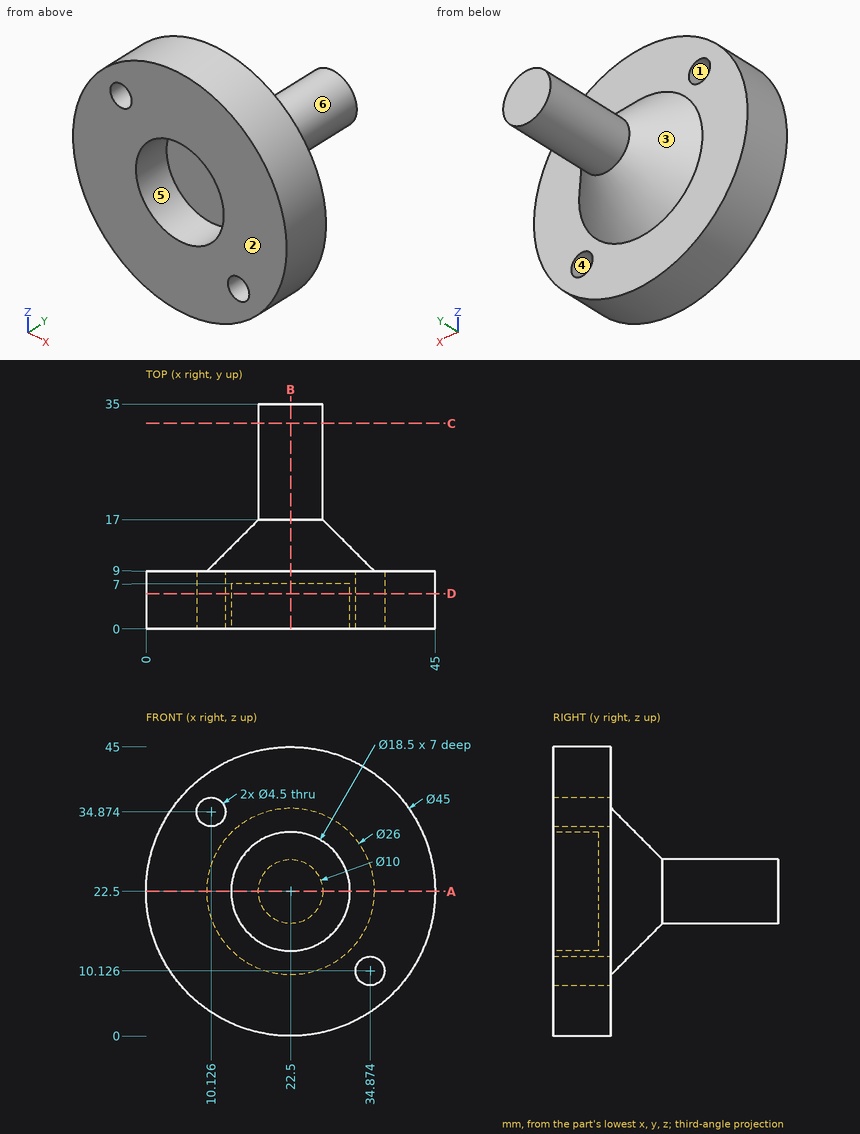
The drawing under review shows one solid part. Ordinate dimensions are in mm from its lowest x, y, z. A direction names the side the tool comes from. Round coordinates to 2 decimals unless told otherwise and drop trailing zeros. Loops run counter-clockwise (first coordinate to the right, second up) from the corner with the lowest first, then second, coordinate; pieces in that order, holes last. Notation, with made-up numbers: (-25.75, 1.25) -> (28.25, 1.25) arc R29 ccw to (28.25, 21.25) -> close; hole circle Ø8 at (-30.5, 70). An arc over 180 degrees is marked (long way). Answer in a Markdown table with one row per item.
1) For pin 1 Ø1 at (x, z) = (21, 9.5) entering from +Y (1 decimal); pin 2 Ø9 at (x, z) = (25, 26) entering from -Y; pin 3 Ø1.5 at (x, y) = (17.5, 17.5) entering from -Z (1 decimal), all flat-tipped, find the tip position at first contact; note any pin that passes through.
Taken from the geometry:
| item | result |
|---|---|
| pin 1 | stops at y = 9.4 |
| pin 2 | stops at y = 7 |
| pin 3 | stops at z = 19.9 |
2) Consider section C-C, the plane y = 32. Write out the cut boundary in (x, z).
Taken from the geometry:
| item | result |
|---|---|
| outline | circle Ø10 at (22.5, 22.5) |
3) Consider section B-B, the plane x = 22.5. Write out the cut boundary in (y, z).
Taken from the geometry:
| item | result |
|---|---|
| outline | (0, 0) -> (9, 0) -> (9, 9.5) -> (17, 17.5) -> (35, 17.5) -> (35, 27.5) -> (17, 27.5) -> (9, 35.5) -> (9, 45) -> (0, 45) -> (0, 31.75) -> (7, 31.75) -> (7, 13.25) -> (0, 13.25) -> close |
4) Draft analysis for pull direction X (two halves, no side actions). For the marked faces 1, 2 and 3, state which applies: pulls with the +X half, pulls with the -X half, needs draft (parallel to the pull), parting line crosses it, or undercut.
Taken from the geometry:
| item | result |
|---|---|
| face 1 | undercut |
| face 2 | needs draft |
| face 3 | parting line crosses it |
5) Consider section D-D, the plane y = 5.5. Count the separate pieces of the cut face and the enclosed holes in it, plus the area to 3 significant figures.
Taken from the geometry:
| item | result |
|---|---|
| separate pieces | 1 |
| enclosed holes | 3 |
| area | 1,290 mm² |
6) Consider section A-A, the plane z = 22.5. Write out the cut boundary in (x, y).
Taken from the geometry:
| item | result |
|---|---|
| outline | (0, 0) -> (13.25, 0) -> (13.25, 7) -> (31.75, 7) -> (31.75, 0) -> (45, 0) -> (45, 9) -> (35.5, 9) -> (27.5, 17) -> (27.5, 35) -> (17.5, 35) -> (17.5, 17) -> (9.5, 9) -> (0, 9) -> close |
7) Tool access review of the marked faces 4, 5 and 6: name each direction out of +Z, -Z, +X, -X, +Y, -Y from which nothing blocks a thin tool from reaching the whole face with its end or side.
Taken from the geometry:
| item | result |
|---|---|
| face 4 | +Y, -Y |
| face 5 | -Y |
| face 6 | +Y |
8) Wall thickness on line 1 along Z through (x, y) = (22.5, 2.75); line 2 along Y through (x, z) = (25.5, 22.5); line 3 along Y through (x, z) = (2.5, 29.5): over which ranges is each line inside the solid? List them lowest first.
Taken from the geometry:
| item | result |
|---|---|
| line 1 | z = 0 to 13.25, 31.75 to 45 |
| line 2 | y = 7 to 35 |
| line 3 | y = 0 to 9 |
